from build123d import *

# Parameters (mm, degrees)
BOSS_EXTRUDE2_DEPTH = 1.5
SKETCH3_R           = 3.5
CUT_EXTRUDE1_DEPTH  = 58.764549458


with BuildPart() as part:
    # Sketch1 → Boss-Extrude2 (new, symmetric)
    with BuildSketch(Plane(origin=(0, 0, 0), x_dir=(1, 0, 0), z_dir=(0, 1, 0))):
        with BuildLine():
            Line((-40, 0), (-40, -16.366130131))
            ThreePointArc((-40, -16.366130131), (-38.348645293, -21.23385064), (-34.076324263, -24.091987854))
            Line((-34.076324263, -24.091987854), (29.923675737, -41.291987854))
            ThreePointArc((29.923675737, -41.291987854), (36.867720508, -39.914775424), (40, -33.566130131))
            Line((40, -33.566130131), (40, 0))
            Line((40, 0), (-40, 0))
        make_face()
        with BuildLine():
            Line((-40, 16.366130131), (-40, 0))
            Line((-40, 0), (40, 0))
            Line((40, 0), (40, 33.566130131))
            ThreePointArc((40, 33.566130131), (36.867720508, 39.914775424), (29.923675737, 41.291987854))
            Line((29.923675737, 41.291987854), (-34.076324263, 24.091987854))
            ThreePointArc((-34.076324263, 24.091987854), (-38.348645293, 21.23385064), (-40, 16.366130131))
        make_face()
    extrude(amount=BOSS_EXTRUDE2_DEPTH, both=True)

    # Sketch3 → Cut-Extrude1 (cut, through all)
    with BuildSketch(Plane(origin=(0, 1.5, 0), x_dir=(1, 0, 0), z_dir=(0, 1, 0))):
        with Locations(Location((22.315405196, 19, 0), (0, 0, 270))):
            Circle(SKETCH3_R)
        with Locations(Location((-28, 12, 0), (0, 0, 270))):
            Circle(SKETCH3_R)
        with Locations(Location((22.315405196, -19, 0), (0, 0, 90))):
            Circle(SKETCH3_R)
        with Locations(Location((-28, -12, 0), (0, 0, 90))):
            Circle(SKETCH3_R)
    extrude(amount=-CUT_EXTRUDE1_DEPTH, mode=Mode.SUBTRACT)


solid = part.part
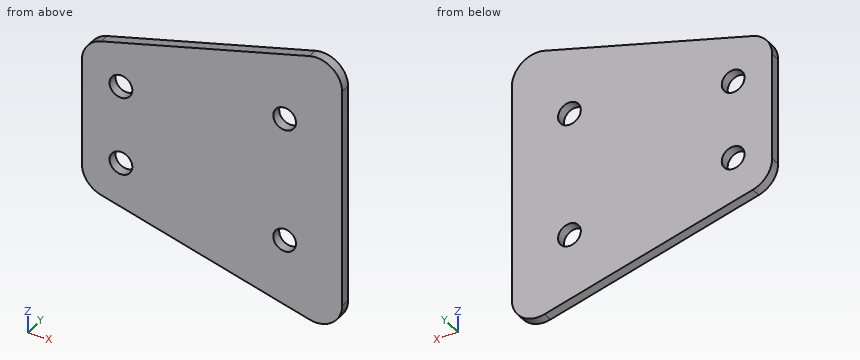
The model under review builds one solid part; all positions refer to its coordinate system, in mm. Round coordinates to 2 decimals unless told otherwise and drop trailing zeros. Loops run counter-clockwise (first coordinate to the right, second up) from the corner with the lowest first, then second, coordinate; pieces in that order, holes last. Notation, with made-up numbers: (6, 18.25) -> (12, 18.25) arc R15 cw to (12, 42.25) -> close; hole circle Ø4 at (53, -13.5). An arc over 180 degrees is marked (long way). One line per question, with ' | ' between items. Start each with the question number.
Item 1: Add section B-B, the plane x = -28. Write out the cut boundary in (y, z) (3 decimals).
Item 2: Add section D-D, the plane z = -19. Write out the cut boundary in (x, y), then the cut area to 3 significant figures.
Item 3: Add section A-A, the plane z = 12. Write out the cut boundary in (x, y), then the cut area to 3 significant figures.
Item 4: Add section C-C, the plane y = -1.05. Write out the cut boundary in (x, z), then the cut area to 3 significant figures.
Item 5: Wall thickness on line 1 along Z through (x, y) = (20.5, -0.9); line 2 along X through (y, z) = (0.7, 12); line 3 along X through (y, z) = (-1.2, -13.5): over which ranges is each line inside the solid? List them lowest first. Write a range as [from, to].
Item 6: For pin 1 (1.5 mm diameter, centred on x = 5.5, y = 0.5, fed in from -Z); pin 2 (1 mm diameter, centred on x = 7, y = 1, fed in from +Z), all flat-tipped, find the tip position at first contact; note any pin that passes through.
Return value:
1) outline: (-1.5, -25.725) -> (1.5, -25.725) -> (1.5, -15.5) -> (-1.5, -15.5) -> close; (-1.5, -8.5) -> (1.5, -8.5) -> (1.5, 8.5) -> (-1.5, 8.5) -> close; (-1.5, 15.5) -> (1.5, 15.5) -> (1.5, 25.725) -> (-1.5, 25.725) -> close
2) outline: (-39.55, -1.5) -> (18.82, -1.5) -> (18.82, 1.5) -> (-39.55, 1.5) -> close; (25.82, -1.5) -> (40, -1.5) -> (40, 1.5) -> (25.82, 1.5) -> close | area: 218 mm2
3) outline: (-40, -1.5) -> (-31.5, -1.5) -> (-31.5, 1.5) -> (-40, 1.5) -> close; (-24.5, -1.5) -> (40, -1.5) -> (40, 1.5) -> (-24.5, 1.5) -> close | area: 219 mm2
4) outline: (-40, -16.37) arc R8 ccw to (-34.08, -24.09) -> (29.92, -41.29) arc R8 ccw to (40, -33.57) -> (40, 33.57) arc R8 ccw to (29.92, 41.29) -> (-34.08, 24.09) arc R8 ccw to (-40, 16.37) -> close; hole circle Ø7 at (-28, -12); hole circle Ø7 at (-28, 12); hole circle Ø7 at (22.32, -19); hole circle Ø7 at (22.32, 19) | area: 5,100 mm2
5) line 1: z = [-38.76, -21.99], [-16.01, 16.01], [21.99, 38.76] | line 2: x = [-40, -31.5], [-24.5, 40] | line 3: x = [-40, -31.16], [-24.84, 40]
6) pin 1: stops at z = -34.93 | pin 2: stops at z = 35.27
